Check sheet for the drawn part. Datum: minimum x, y, z corner. Units: mm. Give positions to 0.01 mm unless a question says otherwise; leave off trailing zeros. Order: outer loops, then holes, each group sorted by start corner. A loop starts at its lowest first (then second) coordinate and runs counter-clockwise, first axis right, second up.
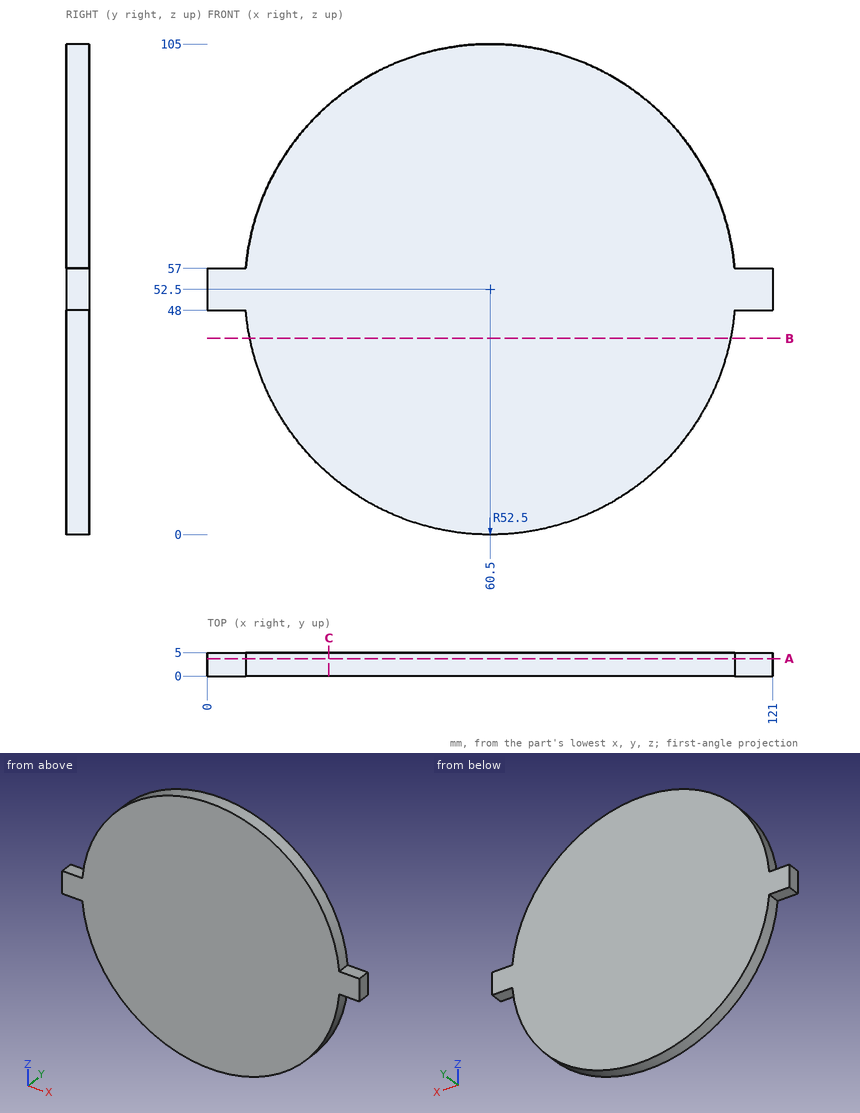
Item 1: Sectioned sample at C-C (x = 26). Enter the section's corners in (y, z).
Reported:
outline: (0, 12.93) - (5, 12.93) - (5, 92.07) - (0, 92.07) - close
Item 2: Sectioned sample at B-B (z = 42). Enter the section's corners in (x, y).
Reported:
outline: (9.06, 0) - (111.94, 0) - (111.94, 5) - (9.06, 5) - close
Item 3: Gauge pin test, flat ends, axial feed: pin 1 (2.5 mm diameter, centred on x = 116.5, y = 3, fed in from +Z); pin 2 (1.5 mm diameter, centred on x = 118.5, y = 1.5, fed in from -Z); pin 3 (1 mm diameter, centred on y = 1.5, z = 62.5, fed in from -X). Record the tip position at first contact, or that the pin passes through.
Reported:
pin 1: stops at z = 57
pin 2: stops at z = 48
pin 3: stops at x = 8.87
Item 4: Scan lines: L1, parallel to Z at x = 88.5, y = 2.45; L2, parallel to Z at x = 44, y = 4.3; L3, parallel to X at y = 4.4, z = 20.5. Record each from-to range of solid material in increasing order.
Reported:
L1: z = 8.09 to 96.91
L2: z = 2.66 to 102.34
L3: x = 18.88 to 102.12
Item 5: Sectioned sample at A-A (y = 3.7). Enter the section's corners in (x, z), and give its area (3 significant figures).
Reported:
outline: (0, 48) - (8.19, 48) arc R52.5 ccw to (112.81, 48) - (121, 48) - (121, 57) - (112.81, 57) arc R52.5 ccw to (8.19, 57) - (0, 57) - close
area: 8,800 mm2
